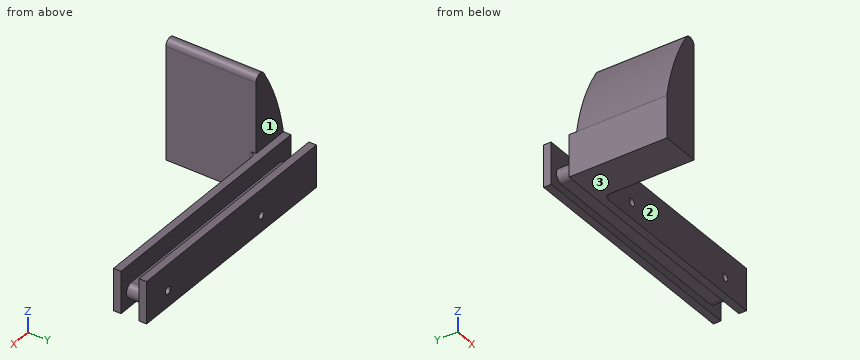
from build123d import *

# Parameters (mm, degrees)
SKETCH2_W           = 101.6
SKETCH2_H           = 17.78
BOSS_EXTRUDE1_DEPTH = 3.175
BOSS_EXTRUDE2_DEPTH = 7.62
BOSS_EXTRUDE3_DEPTH = 38.1
FILLET1_R           = 2.54
FILLET2_R           = 2.54
SKETCH5_R           = 1.524
CUT_EXTRUDE1_DEPTH  = 14.97


with BuildPart() as part:
    # Sketch2 → Boss-Extrude1 (new body)
    with BuildSketch(Plane(origin=(0, 0, 0), x_dir=(1, 0, 0), z_dir=(0, 1, 0))):
        with Locations((50.8, 8.89)):
            Rectangle(SKETCH2_W, SKETCH2_H)
    boss_extrude1 = extrude(amount=BOSS_EXTRUDE1_DEPTH)

    # Sketch3 → Boss-Extrude2 (add)
    with BuildSketch(Plane.XZ):
        with BuildLine():
            Line((95.25, -14.351), (6.35, -14.351))
            ThreePointArc((6.35, -14.351), (3.175, -11.176), (6.35, -8.001))
            Line((6.35, -8.001), (95.25, -8.001))
            ThreePointArc((95.25, -8.001), (98.425, -11.176), (95.25, -14.351))
        make_face()
    extrude(amount=BOSS_EXTRUDE2_DEPTH)

    # Mirror1: Boss-Extrude1 across plane
    add(boss_extrude1.mirror(Plane(origin=(0, -3.81, 0), x_dir=(0, 0, 1), z_dir=(0, -1, 0))))

    # Sketch4 → Boss-Extrude3 (add)
    with BuildSketch(Plane.XZ.offset(10.795)):
        with BuildLine():
            Line((0, -17.78), (16.393849753, -17.78))
            Line((16.393849753, -17.78), (16.393849753, 0))
            Line((16.393849753, 0), (16.393849753, 38.1))
            ThreePointArc((16.393849753, 38.1), (5.909394782, 20.034289362), (0, 0))
            Line((0, 0), (0, -17.78))
        make_face()
    extrude(amount=BOSS_EXTRUDE3_DEPTH)

    # Fillet1
    fillet1_edges = [part.edges().sort_by_distance(p)[0] for p in [
        (16.393849753, -10.795, -8.89),
    ]]
    fillet(fillet1_edges, radius=FILLET1_R)

    # Fillet2
    fillet2_edges = [part.edges().sort_by_distance(p)[0] for p in [
        (16.393849753, -29.845, 38.1),
    ]]
    fillet(fillet2_edges, radius=FILLET2_R)

    # Sketch5 → Cut-Extrude1 (cut, through all)
    with BuildSketch(Plane(origin=(0, -10.795, 0), x_dir=(-1, 0, 0), z_dir=(0, -1, 0))):
        with Locations((-88.9, 10.922)):
            Circle(SKETCH5_R)
        with Locations((-33.02, 10.922)):
            Circle(SKETCH5_R)
    extrude(amount=-CUT_EXTRUDE1_DEPTH, mode=Mode.SUBTRACT)


solid = part.part
Input: part model. Units: mm. Frame: model coordinates. Face numbers are marked on the shaded views. A direction names the side the tool comes from. Coordinates: 2 decimals unless noted, no trailing zeros. Loops run counter-clockwise (first coordinate to the right, second up) from the corner with the lowest first, then second, coordinate; pieces in that order, holes last. Notation, with made-up numbers: (51, -30.5) -> (88, -30.5) arc R21 ccw to (88, -4.5) -> close; hole circle Ø5 at (47.5, 67). An arc over 180 degrees is marked (long way). Write each question's results on one line, items separated by ' | '. Start each with the question number.
Q1. Section B-B, the plane y = -16.5. Return the cut outline in (x, z), plus the area to 3 significant figures.
Q2. Section C-C, the plane x = 56. Return the cut outline in (y, z) (3 decimals), plus the area to 3 significant figures.
Q3. Pin query (flat end, axial travel): pin 1 (6.5 mm diameter, centred on x = 47, y = -10.5, fed in from +Z); pin 2 (14 mm diameter, centred on x = 61.5, z = -11.5, fed in from -Y) (3 decimals); pin 3 (8 mm diameter, centred on x = 21.5, z = 2, fed in from -Y). Return the tip coordinate at first contact, or that it passes through.
Q4. Ray query, line 1 (Z direction, x = 88.9, y = -6.5); line 2 (Y direction, x = 41, z = -0.5) (3 decimals); line 3 (Y direction, x = 9, z = -6.5) (3 decimals). Return the intervals inside material, ascending. Write a range as from..to.
Q5. Section D-D, the plane z = 18. Return the cut outline in (x, y) (3 decimals).
Q6. Reachability of the marked faces 1, 2 and 3 from +Z, -Z, +X, -X, +Y, -Y: full face, straight path, thin tool, end or side. Return the list, or none.
Q7. Section A-A, the plane x = 33.02. Return the cut outline in (y, z) (3 decimals).
Found:
1) outline: (0, -17.78) -> (16.39, -17.78) -> (16.39, 29.86) arc R2.54 ccw to (11.69, 31.19) arc R87.6 ccw to (0, 0) -> close | area: 660 mm2
2) outline: (-10.795, -17.78) -> (-7.62, -17.78) -> (-7.62, -14.351) -> (0, -14.351) -> (0, -17.78) -> (3.175, -17.78) -> (3.175, 0) -> (0, 0) -> (0, -8.001) -> (-7.62, -8.001) -> (-7.62, 0) -> (-10.795, 0) -> close | area: 161 mm2
3) pin 1: z = 0 | pin 2: y = -10.795 | pin 3: y = -10.96
4) line 1: -14.35..-12.45, -9.4..-8 | line 2: -10.795..-7.62, 0..3.175 | line 3: -48.895..-7.62, 0..3.175
5) outline: (5.064, -48.895) -> (16.394, -48.895) -> (16.394, -10.795) -> (5.064, -10.795) -> close
6) face 1: +Z, +X, -X, +Y | face 2: +Z, -Z, +X, -Y | face 3: -Z, +X, -X, +Y, -Y
7) outline: (-10.795, -17.78) -> (-7.62, -17.78) -> (-7.62, -14.351) -> (0, -14.351) -> (0, -17.78) -> (3.175, -17.78) -> (3.175, -12.446) -> (-10.795, -12.446) -> close; (-10.795, -9.398) -> (3.175, -9.398) -> (3.175, 0) -> (0, 0) -> (0, -8.001) -> (-7.62, -8.001) -> (-7.62, 0) -> (-10.795, 0) -> close
